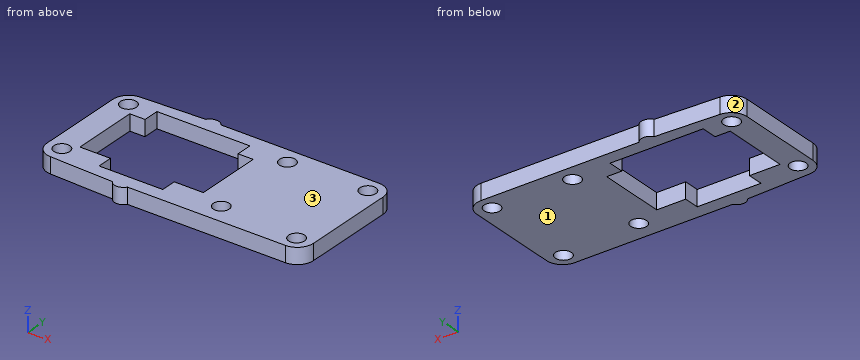
```python
from build123d import *

# Parameters (mm, degrees)
ESQUISSE1_R               = 1.5
T_LE_DE_BASE_PLI_E1_DEPTH = 3
ESQUISSE6_R               = 1.5
ENL_V_MAT_EXTRU_2_DEPTH   = 10


# Sheet-metal steps are written as plain solids
with BuildPart() as part:
    # Esquisse1 → Tôle de base pliée1 (new body)
    with BuildSketch(Plane.XY):
        with BuildLine():
            Line((737.593549902, 733.8762623), (737.593549902, 716.2762623))
            ThreePointArc((737.593549902, 716.2762623), (736.714870246, 714.154941957), (734.593549902, 713.2762623))
            Line((734.593549902, 713.2762623), (704.870597735, 713.2762623))
            ThreePointArc((704.870597735, 713.2762623), (703.450597735, 712.510086472), (702.030597735, 713.2762623))
            Line((702.030597735, 713.2762623), (690.023398786, 713.757541233))
            ThreePointArc((690.023398786, 713.757541233), (687.980166748, 714.67672778), (687.143549902, 716.755134219))
            Line((687.143549902, 716.755134219), (687.143549902, 733.397390382))
            ThreePointArc((687.143549902, 733.397390382), (687.980166748, 735.475796821), (690.023398786, 736.394983368))
            Line((690.023398786, 736.394983368), (702.030597735, 736.8762623))
            ThreePointArc((702.030597735, 736.8762623), (703.450597735, 737.642438129), (704.870597735, 736.8762623))
            Line((704.870597735, 736.8762623), (734.593549902, 736.8762623))
            ThreePointArc((734.593549902, 736.8762623), (736.714870246, 735.997582644), (737.593549902, 733.8762623))
        make_face()
        with Locations((689.943549902, 716.7762623)):
            Circle(ESQUISSE1_R, mode=Mode.SUBTRACT)
        with Locations((734.593549902, 716.0762623)):
            Circle(ESQUISSE1_R, mode=Mode.SUBTRACT)
        with Locations((734.593549902, 734.0762623)):
            Circle(ESQUISSE1_R, mode=Mode.SUBTRACT)
        Polygon((694.693549902, 734.3762623), (712.193549902, 734.3762623), (712.193549902, 731.3762623), (715.043549902, 731.3762623), (715.043549902, 718.7762623), (709.593549902, 718.7762623), (709.593549902, 715.8762623), (697.593549902, 715.8762623), (697.593549902, 718.7762623), (691.843549902, 718.7762623), (691.843549902, 731.3762623), (694.693549902, 731.3762623), align=None, mode=Mode.SUBTRACT)
    extrude(amount=-T_LE_DE_BASE_PLI_E1_DEPTH)

    # Esquisse6 → Enlèv. mat.-Extru.2 (cut)
    with BuildSketch(Plane(origin=(0, 0, -3), x_dir=(-1, 0, 0), z_dir=(0, 0, -1))):
        with Locations((-719.693549902, 733.768635687)):
            Circle(ESQUISSE6_R)
        with Locations((-719.693549902, 717.068635687)):
            Circle(ESQUISSE6_R)
        with Locations((-689.943549902, 733.563854452)):
            Circle(ESQUISSE6_R)
    extrude(amount=-ENL_V_MAT_EXTRU_2_DEPTH, mode=Mode.SUBTRACT)


solid = part.part
```
Here's how the part is built. I have some questions about the finished solid (model axes, mm). Face numbers are marked on the shaded views. Coordinates: 2 decimals unless noted, no trailing zeros. Order: outer loops, then holes, each group sorted by start corner. A loop starts at its lowest first (then second) coordinate and runs counter-clockwise, first axis right, second up.
Item 1: I need wall thicknesses on probe 1 along Y at (x, z) = (690, -0.5); probe 2 along Y at (x, z) = (720.5, -2.2); probe 3 along X at (y, z) = (732.5, -1.8). Which ranges of each line are inside material? Lowest first, please.
Response values:
probe 1: y = 713.76 to 715.28, 718.28 to 732.06, 735.06 to 736.39
probe 2: y = 713.28 to 715.8, 718.33 to 732.5, 735.03 to 736.88
probe 3: x = 687.14 to 688.89, 691 to 694.69, 712.19 to 718.89, 720.49 to 737.59
Item 2: I'm going to push flat-ended pins straight in: pin 1 Ø1.5 at (x, z) = (706, -1.5) entering from -Y; pin 2 Ø1.5 at (x, z) = (713, -1) entering from +Y. Where does each tip first touch, or does it pass through?
Response values:
pin 1: stops at y = 713.28
pin 2: stops at y = 736.88
Item 3: If we section it at C-C, the plane z = -2.1: Give the number of separate pieces and of enclosed holes in the cut face, then the cut area to 3 significant figures.
Response values:
separate pieces: 1
enclosed holes: 7
area: 755 mm2
Item 4: Thinking about a two-plate mould opening in Z: for the marked faces 1, 2 and 3, which applies, pulls with the +Z half, pulls with the -Z half, needs draft (parallel to the pull), parting line crosses it, or undercut?
Response values:
face 1: pulls with the -Z half
face 2: needs draft
face 3: pulls with the +Z half
Item 5: If we section it at D-D, the plane x = 727: List the corners of the cut face in (y, z) for me.
Response values:
outline: (713.28, -3) - (736.88, -3) - (736.88, 0) - (713.28, 0) - close
Item 6: If we section it at A-A, the plane y = 730: List the corners of the cut face in (x, z) for me, then the cut area to 4 significant figures.
Response values:
outline: (687.14, -3) - (691.84, -3) - (691.84, 0) - (687.14, 0) - close; (715.04, -3) - (737.59, -3) - (737.59, 0) - (715.04, 0) - close
area: 81.75 mm2
Item 7: If we section it at B-B, the plane x = 707: List the corners of the cut face in (y, z) for me, then the cut area to 3 significant figures.
Response values:
outline: (713.28, -3) - (715.88, -3) - (715.88, 0) - (713.28, 0) - close; (734.38, -3) - (736.88, -3) - (736.88, 0) - (734.38, 0) - close
area: 15.3 mm2
